from build123d import *

# Parameters (mm, degrees)
SKETCH2_W           = 400
SKETCH2_H           = 20
SKETCH2_R           = 5
BOSS_EXTRUDE1_DEPTH = 10
FILLET1_RADIUS      = 10
FILLET1_LENGTH      = 10


with BuildPart() as part:
    # Sketch2 → Boss-Extrude1 (new body)
    with BuildSketch(Plane(origin=(0, 0, 0), x_dir=(1, 0, 0), z_dir=(0, 1, 0))):
        with Locations((89.044360902, -13.673273177)):
            Rectangle(SKETCH2_W, SKETCH2_H)
        with Locations(Location((272.933671002, -13.673273177, 0), (0, 0, 270))):
            Circle(SKETCH2_R, mode=Mode.SUBTRACT)
    extrude(amount=BOSS_EXTRUDE1_DEPTH)

    # Fillet1: full round fillet: the end face becomes a half cylinder, R = half its width
    fillet1_face = Plane((289.044360902, 5, 13.673273177), x_dir=(0, 1, 0), z_dir=(1, 0, 0))  # on the end face: x along it, z out of the body
    fillet1_slab = fillet1_face.offset(-FILLET1_RADIUS / 2) * Box(FILLET1_LENGTH, 2 * FILLET1_RADIUS, FILLET1_RADIUS, mode=Mode.PRIVATE)  # the body's end, R deep
    fillet1_round = Plane((279.044360902, 5, 13.673273177), x_dir=(1, 0, 0), z_dir=(0, 1, 0)) * Cylinder(FILLET1_RADIUS, FILLET1_LENGTH, mode=Mode.PRIVATE)  # its axis R under the face
    add(fillet1_slab - fillet1_round, mode=Mode.SUBTRACT)


solid = part.part
Here's how the part is built. I have some questions about the finished solid (model axes, mm). Round coordinates to 2 decimals unless told otherwise and drop trailing zeros. Loops run counter-clockwise (first coordinate to the right, second up) from the corner with the lowest first, then second, coordinate; pieces in that order, holes last. Notation, with made-up numbers: (4, 37.5) -> (48, 37.5) arc R15 cw to (48, 56.5) -> close; hole circle Ø3 at (52.5, 53). An arc over 180 degrees is marked (long way). Write each question's results on one line, items separated by ' | '.
(1) If we section it at A-A, the plane z = 15: List the corners of the cut face in (x, y) for me.
Worked answers:
outline: (-110.96, 0) -> (268.11, 0) -> (268.11, 10) -> (-110.96, 10) -> close; (277.75, 0) -> (288.96, 0) -> (288.96, 10) -> (277.75, 10) -> close
(2) If we section it at B-B, the plane y = 7.25: List the corners of the cut face in (x, z) for me.
Worked answers:
outline: (-110.96, 3.67) -> (279.04, 3.67) arc R10 ccw to (279.04, 23.67) -> (-110.96, 23.67) -> close; hole circle Ø10 at (272.93, 13.67)
(3) We'd pull the mould along Z, two halves only. Please class faces 1 (the face through (277.15, 4.93, 16.36)), 2 (the face through (81, 5, 3.673)), 3 (the face through (86, 10, 14)): released by +Z, released by -Z, zero draft, split by the parting line, or undercut.
Worked answers:
face 1: undercut | face 2: released by -Z | face 3: zero draft
(4) If I drill on L1, parallel to X at y = 8.25, z = 14; L2, parallel to X at y = 7.25, z = 15; L3, parallel to X at y = 4.75, z = 8.5, over which ranges is the centre line in solid material (lowest first)?
Worked answers:
L1: -110.96 to 267.94, 277.92 to 289.04 | L2: -110.96 to 268.11, 277.75 to 288.96 | L3: -110.96 to 287.6
(5) For P1, Ø6, axis at x = 272.93, z = 13.67, coming from the +Y side; P2, Ø1, axis at y = 5.5, z = 15.5, coming from the +X side, each with a flat end and sliding along its axis, tell me the tip position at first contact or that it passes through.
Worked answers:
P1: through | P2: x = 288.96
